```python
from build123d import *

# Parameters (mm, degrees)
SKIZZE1_W                            = 180
SKIZZE1_H                            = 50
AUFSATZ_LINEAR_AUSTRAGEN1_DEPTH      = 20
SKIZZE2_R                            = 2.75
SCHNITT_LINEAR_AUSTRAGEN1_DEPTH      = 40
SKIZZE3_R                            = 5
SCHNITT_LINEAR_AUSTRAGEN2_DEPTH      = 6
F_4_2_4_2_DURCHMESSER_BOHRUNG1_D     = 4.2
F_4_2_4_2_DURCHMESSER_BOHRUNG1_DEPTH = 34
F_4_2_4_2_DURCHMESSER_BOHRUNG1_TIP   = 1.2618073


with BuildPart() as part:
    # Skizze1 → Aufsatz-Linear austragen1 (new body)
    with BuildSketch(Plane.XY):
        with Locations((0, 25)):
            Rectangle(SKIZZE1_W, SKIZZE1_H)
    extrude(amount=AUFSATZ_LINEAR_AUSTRAGEN1_DEPTH)

    # Skizze2 → Schnitt-Linear austragen1 (cut)
    with BuildSketch(Plane.XY.offset(20)):
        with Locations((34, 9)):
            Circle(SKIZZE2_R)
        with Locations((70, 9)):
            Circle(SKIZZE2_R)
        with Locations(Location((70, 41, 0), (0, 0, 180))):
            Circle(SKIZZE2_R)
        with Locations(Location((34, 41, 0), (0, 0, 180))):
            Circle(SKIZZE2_R)
        with Locations(Location((-34, 9, 0), (0, 0, 180))):
            Circle(SKIZZE2_R)
        with Locations(Location((-70, 9, 0), (0, 0, 180))):
            Circle(SKIZZE2_R)
        with Locations((-70, 41)):
            Circle(SKIZZE2_R)
        with Locations((-34, 41)):
            Circle(SKIZZE2_R)
    extrude(amount=-SCHNITT_LINEAR_AUSTRAGEN1_DEPTH, mode=Mode.SUBTRACT)

    # Skizze3 → Schnitt-Linear austragen2 (cut)
    with BuildSketch(Plane.XY):
        with Locations((-70, 41)):
            Circle(SKIZZE3_R)
        with Locations((-34, 41)):
            Circle(SKIZZE3_R)
        with Locations((34, 41)):
            Circle(SKIZZE3_R)
        with Locations((70, 41)):
            Circle(SKIZZE3_R)
        with Locations((70, 9)):
            Circle(SKIZZE3_R)
        with Locations((34, 9)):
            Circle(SKIZZE3_R)
        with Locations((-34, 9)):
            Circle(SKIZZE3_R)
        with Locations((-70, 9)):
            Circle(SKIZZE3_R)
    extrude(amount=SCHNITT_LINEAR_AUSTRAGEN2_DEPTH, mode=Mode.SUBTRACT)

    # Ø4.2 (4.2) Durchmesser Bohrung1
    with Locations(Plane(origin=(0, 0, 0), x_dir=(-1, 0, 0), z_dir=(0, 0, -1))):
        with Locations((-22, 9), (82, 41), (22, 41), (82, 9), (22, 9), (-82, 9), (-82, 41), (-22, 41)):
            Hole(F_4_2_4_2_DURCHMESSER_BOHRUNG1_D / 2, depth=F_4_2_4_2_DURCHMESSER_BOHRUNG1_DEPTH)
            with Locations((0, 0, -(F_4_2_4_2_DURCHMESSER_BOHRUNG1_DEPTH + F_4_2_4_2_DURCHMESSER_BOHRUNG1_TIP / 2))):  # 118° drill point
                Cone(0, F_4_2_4_2_DURCHMESSER_BOHRUNG1_D / 2, F_4_2_4_2_DURCHMESSER_BOHRUNG1_TIP, mode=Mode.SUBTRACT)


solid = part.part
```
Input: part model. Units: mm. Frame: model coordinates. A direction names the side the tool comes from. Round coordinates to 2 decimals unless told otherwise and drop trailing zeros. Loops run counter-clockwise (first coordinate to the right, second up) from the corner with the lowest first, then second, coordinate; pieces in that order, holes last. Notation, with made-up numbers: (1.25, -29.5) -> (20.25, -29.5) arc R25 cw to (20.25, -5.5) -> close; hole circle Ø8 at (1, 57). An arc over 180 degrees is marked (long way). One line per item, written item: value.
(1) Material intervals for line 1 (Y direction, x = 70, z = 2.45); line 2 (Y direction, x = -22, z = 9.25); line 3 (X direction, y = 43.5, z = 7.75), sorted ascending. Write a range as [from, to].
Geometry check:
line 1: [0, 4], [14, 36], [46, 50]
line 2: [0, 6.9], [11.1, 38.9], [43.1, 50]
line 3: [-90, -71.15], [-68.85, -35.15], [-32.85, 32.85], [35.15, 68.85], [71.15, 90]
(2) Mould query, pull axis Y, two halves, no side actions, for faces 3 (the face through (-67.8, 38.8, 6)), 4 (the face through (-90, 25, 10)), 5 (the face through (-1, 50, 10)). Classes: pulls with the +Y half, pulls with the -Y half, needs draft (parallel to the pull), parting line crosses it, or undercut.
Geometry check:
face 3: undercut
face 4: needs draft
face 5: pulls with the +Y half
(3) Set-up query: faces 1 (the face through (22.969, 39.137, 10.14)), 2 (the face through (-31.8, 38.8, 6)). Return all of +Z, -Z, +X, -X, +Y, -Y with unobstructed straight access to the full face (end or side cutting, diameter ignored); none if empty.
Geometry check:
face 1: +Z, -Z
face 2: -Z
(4) Section B-B (z = 9.5). Give the number of separate pieces and of enclosed holes in the cut face, plus the area to 3 significant figures.
Geometry check:
separate pieces: 1
enclosed holes: 16
area: 8,700 mm2
(5) Pin query (flat end, axial travel): pin 1 (9 mm diameter, centred on x = 70, y = 41, fed in from -Z); pin 2 (3.5 mm diameter, centred on x = -34, y = 9, fed in from -Z). Return the tip coordinate at first contact, or that it passes through.
Geometry check:
pin 1: z = 6
pin 2: through
(6) Section D-D (x = 69). Return the cut outline in (y, z), plus the area to 3 significant figures.
Geometry check:
outline: (0, 0) -> (4.1, 0) -> (4.1, 6) -> (6.44, 6) -> (6.44, 20) -> (0, 20) -> close; (11.56, 6) -> (13.9, 6) -> (13.9, 0) -> (36.1, 0) -> (36.1, 6) -> (38.44, 6) -> (38.44, 20) -> (11.56, 20) -> close; (43.56, 6) -> (45.9, 6) -> (45.9, 0) -> (50, 0) -> (50, 20) -> (43.56, 20) -> close
area: 739 mm2
(7) Section A-A (x = -70). Return the cut outline in (y, z).
Geometry check:
outline: (0, 0) -> (4, 0) -> (4, 6) -> (6.25, 6) -> (6.25, 20) -> (0, 20) -> close; (11.75, 6) -> (14, 6) -> (14, 0) -> (36, 0) -> (36, 6) -> (38.25, 6) -> (38.25, 20) -> (11.75, 20) -> close; (43.75, 6) -> (46, 6) -> (46, 0) -> (50, 0) -> (50, 20) -> (43.75, 20) -> close
